Source: CAD feature listing. Evaluate the final solid. Frame: model axes, mm. Face numbers are marked on the shaded views. A direction names the side the tool comes from. Coordinates: 2 decimals unless noted, no trailing zeros. Order: outer loops, then holes, each group sorted by start corner. A loop starts at its lowest first (then second) coordinate and runs counter-clockwise, first axis right, second up. Notation, with made-up numbers: (7.5, 87) - (50.5, 87) arc R5 cw to (50.5, 94) - close; hole circle Ø9 at (28, 12). An arc over 180 degrees is marked (long way). One line per question, with ' | ' between items. Start each with the question number.
(1) Draft query along Y for the marked faces 3, 4, 5 and 6. Return one class per face: +Y half, -Y half, draft (parallel to the pull), parting line (faces both ways), or undercut.
(2) Contact query for a flat-ended pin moving along its axis: P1, Ø3, axis at y = 17.5, z = 4, coming from the -X side. Output: stop coordinate, or through.
(3) Line query: line 1 along Y through (x, z) = (12.25, 2.5); line 2 along X through (y, z) = (15.25, 0.4); line 3 along X through (y, z) = (17, 4.4). Output: solid intervals per line, ascending.
(4) Section B-B (z = 3.75). Return the cut outline in (x, y), then the cut area to 3 significant figures.
(5) Section A-A (x = 4.5). Return the cut outline in (y, z), then the cut area to 3 significant figures.
(6) Section C-C (y = 15). Return the cut outline in (x, z), then the cut area to 3 significant figures.
(7) Access query for the marked faces 1 and 2. Directions: +Z, -Z, +X, -X, +Y, -Y. A direction counts if a zero-diameter tool reaches every point of the face in a straight line with its end or side. Return the directions, or none.
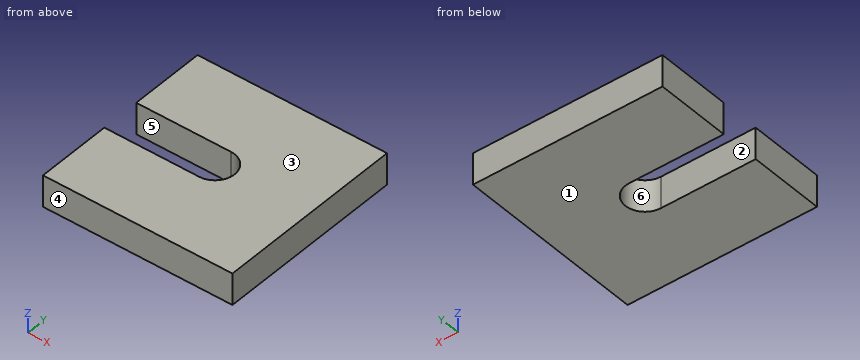
from build123d import *

# Parameters (mm, degrees)
BOSS_EXTRUDE1_DEPTH = 5


with BuildPart() as part:
    # Sketch1 → Boss-Extrude1 (new body)
    with BuildSketch(Plane.XY):
        with BuildLine():
            Line((15, 18.1), (0, 18.1))
            Line((0, 18.1), (0, 30))
            Line((0, 30), (30, 30))
            Line((30, 30), (30, 0))
            Line((30, 0), (0, 0))
            Line((0, 0), (0, 11.9))
            Line((0, 11.9), (15, 11.9))
            ThreePointArc((15, 11.9), (18.1, 15), (15, 18.1))
        make_face()
    extrude(amount=BOSS_EXTRUDE1_DEPTH)


solid = part.part
Response values:
1) face 3: draft | face 4: -Y half | face 5: undercut | face 6: undercut
2) P1: stops at x = 0
3) line 1: y = 0 to 11.9, 18.1 to 30 | line 2: x = 18.09 to 30 | line 3: x = 17.37 to 30
4) outline: (0, 0) - (30, 0) - (30, 30) - (0, 30) - (0, 18.1) - (15, 18.1) arc R3.1 cw to (15, 11.9) - (0, 11.9) - close | area: 792 mm²
5) outline: (0, 0) - (11.9, 0) - (11.9, 5) - (0, 5) - close; (18.1, 0) - (30, 0) - (30, 5) - (18.1, 5) - close | area: 119 mm²
6) outline: (18.1, 0) - (30, 0) - (30, 5) - (18.1, 5) - close | area: 59.5 mm²
7) face 1: -Z, +X, -X, +Y, -Y | face 2: +Z, -Z, -X
